Autodesk Inventor part; units mm, degrees
ref_plane "YZ Plane" through (0, 0, 0) normal (1, 0, 0) x (0, 1, 0)
ref_plane "XZ Plane" through (0, 0, 0) normal (0, 1, 0) x (-1, 0, 0)
ref_plane "XY Plane" through (0, 0, 0) normal (0, 0, 1) x (1, 0, 0)
sketch "Sketch1" plane through (0, 0, 0) normal (0, 1, 0) x (-1, 0, 0)
  line L0 (0, 0) -> (61, 0)
  line L1 (61, 0) -> (61, -77)
  line L2 (61, -77) -> (0, -77)
  line L3 (0, -77) -> (0, 0)
  line L4 (61, -35) -> (54, -35) construction
  line L5 (54, -35) -> (54, -42) construction
  line L6 (54, -42) -> (61, -42) construction
  line L7 (61, -42) -> (61, -35) construction
  line L8 (30.5, 0) -> (30.5, -77) construction
  line L9 (57.5, -35) -> (57.5, -42) construction
  line L10 (61, -38.5) -> (54, -38.5) construction
  circle A0 centre (57.5, -38.5) radius 1.8
  circle A1 centre (3.5, -38.5) radius 1.8
  dimension "d0" = 61
  dimension "d1" = 77
  dimension "d2" = 7
  dimension "d3" = 7
  dimension "d4" = 35
  dimension "d5" = 3.6
extrude "Extrusion1" add sketch "Sketch1" along normal blind 4
sketch "Sketch2" plane through (0, 4, 0) normal (0, 1, 0) x (1, 0, 0)
  line L0 (-61, 77) -> (-61, 0)
  line L1 (-61, 0) -> (0, 0)
  line L2 (0, 0) -> (0, 8)
  line L3 (0, 8) -> (-61, 8)
  line L4 (-61, 8) -> (-61, 0)
  line L5 (-61, 0) -> (-53, 0)
  line L6 (-53, 0) -> (-53, 16)
  line L7 (-53, 16) -> (-61, 16)
  line L8 (-61, 16) -> (-61, 0)
  line L9 (-61, 0) -> (0, 0)
  line L10 (0, 0) -> (-8, 0)
  line L11 (-8, 0) -> (-8, 16)
  line L12 (-8, 16) -> (0, 16)
  line L13 (0, 16) -> (0, 0)
  line L14 (-61, 38.5) -> (0, 38.5) construction
  line L15 (0, 0) -> (0, 77)
  line L16 (-61, 77) -> (0, 77)
  line L17 (0, 77) -> (0, 69)
  line L18 (0, 69) -> (-61, 69)
  line L19 (-61, 69) -> (-61, 77)
  line L20 (-61, 77) -> (-53, 77)
  line L21 (-53, 77) -> (-53, 61)
  line L22 (-53, 61) -> (-61, 61)
  line L23 (-61, 61) -> (-61, 77)
  line L24 (-61, 77) -> (0, 77)
  line L25 (0, 77) -> (-8, 77)
  line L26 (-8, 77) -> (-8, 61)
  line L27 (-8, 61) -> (0, 61)
  line L28 (0, 61) -> (0, 77)
  point P0 (-8, 69)
  point P1 (0, 61)
  point P2 (-53, 69)
  point P3 (-8, 8)
  point P4 (-53, 8)
  dimension "d8" = 8
  dimension "d9" = 8
  dimension "d10" = 16
  dimension "d11" = 8
  dimension "d12" = 16
extrude "Extrusion2" add sketch "Sketch2" along normal blind 6 contours L16 L21 L18 L0 | L18 L21 L22 L0 | L16 L26 L18 L21 | L16 L15 L18 L26 | L7 L6 L3 L0 | L18 L15 L27 L26 | L3 L6 L1 L0 | L3 L11 L1 L6 | L11 L12 L13 L3 | L3 L2 L1 L11
sketch "Sketch3" plane through (0, 4, 0) normal (0, 1, 0) x (1, 0, 0)
  line L0 (-51.5, 8) -> (-9.5, 8) construction
  line L1 (-9.5, 8) -> (-9.5, 69) construction
  line L2 (-9.5, 69) -> (-51.5, 69) construction
  line L3 (-51.5, 69) -> (-51.5, 8) construction
  line L4 (-61, 61) -> (-61, 16)
  line L5 (-61, 0) -> (0, 0)
  line L6 (-9.5, 69) -> (-21.5, 69)
  line L7 (-21.5, 69) -> (-21.5, 39)
  line L8 (-21.5, 39) -> (-9.5, 39)
  line L9 (-9.5, 39) -> (-9.5, 69)
  line L10 (-9.5, 66) -> (-9.5, 54)
  line L11 (-9.5, 69) -> (-29.5, 69)
  line L12 (-29.5, 69) -> (-29.5, 57)
  line L13 (-29.5, 57) -> (-9.5, 57)
  line L14 (-9.5, 57) -> (-9.5, 69)
  point P0 (-21.5, 57)
  dimension "d15" = 42
  dimension "d16" = 61
  dimension "d17" = 9.5
  dimension "d18" = 8
  dimension "d19" = 12
  dimension "d20" = 30
  dimension "d25" = 20
  dimension "d26" = 12
extrude "Extrusion3" cut sketch "Sketch3" against normal through all
properties part number "ESPLid"
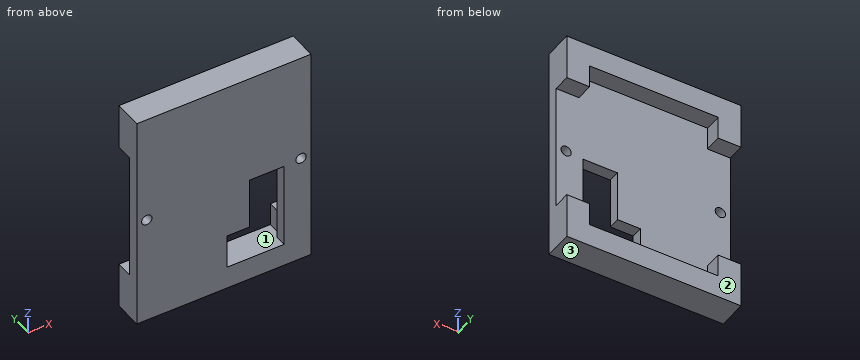
Could you check a few things on this model? Use its own coordinates, in mm. Face numbers are marked on the shaded views. Give positions to 0.01 mm unless a question says otherwise; leave off trailing zeros. Order: outer loops, then holes, each group sorted by start corner. A loop starts at its lowest first (then second) coordinate and runs counter-clockwise, first axis right, second up. Notation, with made-up numbers: (84.5, 20.25) -> (132.5, 20.25) arc R22 cw to (132.5, 33.25) -> close; hole circle Ø9 at (34.25, -22). An arc over 180 degrees is marked (long way). Return JSON: item names as keys, results as strings.
1. Imagine slicing it at C-C on x = -10.5. List the corners of the cut face in (y, z) for me, then the cut area to 3 significant figures.
Answer list:
{"outline": "(0, -77) -> (10, -77) -> (10, -69) -> (0, -69) -> close; (0, -39) -> (4, -39) -> (4, -8) -> (10, -8) -> (10, 0) -> (0, 0) -> close", "area": "284 mm2"}
2. Imagine slicing it at D-D on y = 3. List the corners of the cut face in (x, z) for me, then the cut area to 3 significant figures.
Answer list:
{"outline": "(-61, -77) -> (0, -77) -> (0, 0) -> (-61, 0) -> close; hole circle Ø3.6 at (-57.5, -38.5); hole (-29.5, -69) -> (-9.5, -69) -> (-9.5, -39) -> (-21.5, -39) -> (-21.5, -57) -> (-29.5, -57) -> close; hole circle Ø3.6 at (-3.5, -38.5)", "area": "4,220 mm2"}
3. For pin 1 Ø5 at (x, z) = (-27.5, -35.5) entering from +Y; pin 2 Ø1.5 at (y, z) = (5, -38) entering from +X, each with a flat end and sliding along its axis, tell me the tip position at first contact or that it passes through.
Answer list:
{"pin 1": "stops at y = 4", "pin 2": "passes through"}
4. Thinking about a two-plate mould opening in Z: for the marked faces 1, 2 and 3, which applies, pulls with the +Z half, pulls with the -Z half, needs draft (parallel to the pull), parting line crosses it, or undercut?
Answer list:
{"face 1": "undercut", "face 2": "needs draft", "face 3": "pulls with the -Z half"}
5. Imagine slicing it at B-B on y = 8.75. List the corners of the cut face in (x, z) for me.
Answer list:
{"outline": "(-61, -77) -> (0, -77) -> (0, -61) -> (-8, -61) -> (-8, -69) -> (-53, -69) -> (-53, -61) -> (-61, -61) -> close; (-61, -16) -> (-53, -16) -> (-53, -8) -> (-8, -8) -> (-8, -16) -> (0, -16) -> (0, 0) -> (-61, 0) -> close"}
6. I need wall thicknesses on line 1 (Z direction, x = -57.5, y = 2.3); line 2 (Z direction, x = -24, y = 8.5); line 3 (X direction, y = 9.5, z = -63.5). Which ranges of each line are inside material? Lowest first, please. Write a range as from..to.
Answer list:
{"line 1": "z = -77..-40.3, -36.7..0", "line 2": "z = -77..-69, -8..0", "line 3": "x = -61..-53, -8..0"}
7. Imagine slicing it at A-A on z = -49. List the corners of the cut face in (x, y) for me.
Answer list:
{"outline": "(-61, 0) -> (-21.5, 0) -> (-21.5, 4) -> (-61, 4) -> close; (-9.5, 0) -> (0, 0) -> (0, 4) -> (-9.5, 4) -> close"}
